Part model, mm, in its own coordinate system. Coordinates: 2 decimals unless noted, no trailing zeros. Loops run counter-clockwise (first coordinate to the right, second up) from the corner with the lowest first, then second, coordinate; pieces in that order, holes last. Notation, with made-up numbers: (52.5, 14.5) - (87.5, 14.5) arc R20 ccw to (87.5, 25.5) - close; hole circle Ø2 at (11.25, -33.75). An arc over 180 degrees is marked (long way). Use a Markdown table: item, result. Add a question column.
1) Band-saw the part on A-A (x = -108.5). Give the cut face in (y, z), plus the area to 3 significant figures.
2) Drop flat-ended pins along their axis: P1, Ø4.5, axis at x = -341.5, y = 9.5, coming from the -Z side; P2, Ø4, axis at x = -273, z = -14.5, coming from the +Y side; P3, Ø1, axis at x = -281.5, y = 10, coming from the -Z side; P4, Ø2, axis at x = -281, y = 7.5, coming from the +Z side. Give the stop position or say it passes through.
3) Probe probe 1 along X at (y, z) = (9.5, -1.05); probe 2 along Y at (x, z) = (-6.5, -1.1); probe 3 along Y at (x, z) = (-31.5, -1.9). List the from-to ranges inside material, lowest first. Write a range as [from, to].
4) Band-saw the part on B-B (x = -191). Give the cut face in (y, z).
from build123d import *

# Parameters (mm, degrees)
SKETCH1_W              = 66
SKETCH1_H              = 4
BOSS_EXTRUDE1_DEPTH    = 19
CUT_EXTRUDE5_START     = -16.909
CUT_EXTRUDE5_OUTLINE_R = 2.5
CUT_EXTRUDE5_DEPTH     = 16.909


# Read off the part's stored shape, not the designer's step: Cut-Extrude5
with BuildPart() as part:
    # Sketch1 → Boss-Extrude1 (new body)
    with BuildSketch(Plane(origin=(0, 0, 0), x_dir=(1, 0, 0), z_dir=(0, 1, 0))):
        with Locations((-33, 2)):
            Rectangle(SKETCH1_W, SKETCH1_H)
        Polygon((-66, 0), (-66, 4), (-348, 16.909), (-348, 12.909), align=None)
    extrude(amount=BOSS_EXTRUDE1_DEPTH)

    # Cut-Extrude5 outline → Cut-Extrude5 (cut)
    with BuildSketch(Plane.XY.offset(CUT_EXTRUDE5_START)):
        with BuildLine():
            ThreePointArc((-348, 9.5), (-346.096194078, 14.096194078), (-341.5, 16))
            Line((-341.5, 16), (-66, 19))
            Line((-66, 19), (-348, 19))
            Line((-348, 19), (-348, 9.5))
        make_face()
        with BuildLine():
            ThreePointArc((-341.5, 3), (-346.096194078, 4.903805922), (-348, 9.5))
            Line((-348, 9.5), (-348, 0))
            Line((-348, 0), (-66, 0))
            Line((-66, 0), (-341.5, 3))
        make_face()
        with BuildLine():
            Line((0, 19), (-66, 19))
            Line((-66, 19), (-6.5, 16))
            ThreePointArc((-6.5, 16), (-1.903805922, 14.096194078), (0, 9.5))
            Line((0, 9.5), (0, 19))
        make_face()
        with BuildLine():
            Line((-6.5, 3), (-66, 0))
            Line((-66, 0), (0, 0))
            Line((0, 0), (0, 9.5))
            ThreePointArc((0, 9.5), (-1.903805922, 4.903805922), (-6.5, 3))
        make_face()
        with Locations((-341.5, 9.5)):
            Circle(CUT_EXTRUDE5_OUTLINE_R)
        with BuildLine():
            Line((-75.5, 12), (-279, 9.5))
            Line((-279, 9.5), (-75.5, 7))
            ThreePointArc((-75.5, 7), (-73, 9.5), (-75.5, 12))
        make_face()
        with Locations((-6.5, 9.5)):
            Circle(CUT_EXTRUDE5_OUTLINE_R)
        with Locations((-31.5, 9.5)):
            Circle(CUT_EXTRUDE5_OUTLINE_R)
        with Locations((-56.5, 9.5)):
            Circle(CUT_EXTRUDE5_OUTLINE_R)
    extrude(amount=CUT_EXTRUDE5_DEPTH, mode=Mode.SUBTRACT)


solid = part.part
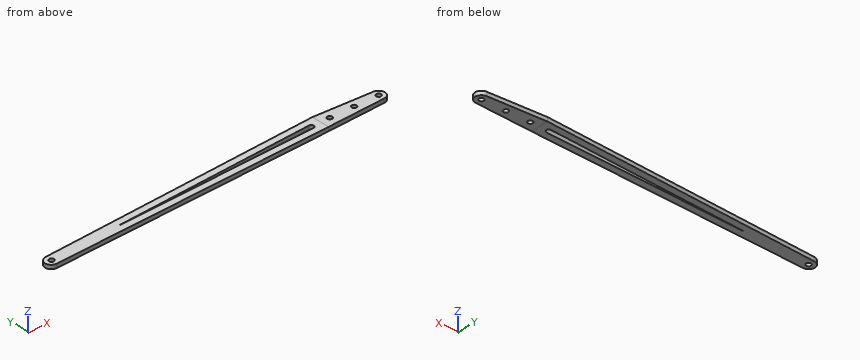
Answer block:
| question | item | result |
|---|---|---|
| 1 | outline | (0.46, -5.95) - (7.41, -5.95) - (7.41, -1.95) - (0.46, -1.95) - close; (11.59, -5.95) - (18.54, -5.95) - (18.54, -1.95) - (11.59, -1.95) - close |
| 1 | area | 55.5 mm2 |
| 2 | P1 | through |
| 2 | P2 | y = 16.76 |
| 2 | P3 | z = -13.89 |
| 2 | P4 | z = -9.8 |
| 3 | probe 1 | [-73, -59], [-54, -34], [-29, -9], [-4, 0] |
| 3 | probe 2 | [3, 7], [12, 16] |
| 3 | probe 3 | [1.74, 7], [12, 17.26] |
| 4 | outline | (1.36, -9.72) - (8.42, -9.72) - (8.42, -5.72) - (1.36, -5.72) - close; (10.58, -9.72) - (17.64, -9.72) - (17.64, -5.72) - (10.58, -5.72) - close |
